Autodesk Inventor part; units mm, degrees
ref_plane "Work Plane1" through (0, 0, 7.9375) normal (0, 0, 1) x (1, 0, 0)
ref_plane "Work Plane2" through (24.3078, 0, 0) normal (1, 0, 0) x (0, 1, 0)
ref_plane "XZ Plane" through (0, 0, 0) normal (0, 1, 0) x (-1, 0, 0)
sketch "Sketch1" plane through (0, 0, 0) normal (0, 0, 1) x (1, 0, 0)
  line L0 (1.9155, 84.5388) -> (46.3655, 84.5388) construction
  line L1 (46.3655, 84.5388) -> (46.3655, 1.9888) construction
  line L2 (46.3655, 1.9888) -> (1.9155, 1.9888) construction
  line L3 (1.9155, 1.9888) -> (1.9155, 84.5388) construction
  line L4 (13.0242, 66.1379) -> (35.273, 66.1379)
  line L5 (13.0242, 66.1379) -> (13.304, 71.2552)
  line L6 (13.304, 71.2552) -> (14.5683, 76.0081)
  line L7 (14.5683, 76.0081) -> (16.9096, 79.3562)
  line L8 (16.9096, 79.3562) -> (20.1875, 81.1824)
  line L9 (20.1875, 81.1824) -> (24.3082, 82.0721)
  line L10 (24.3082, 82.0721) -> (24.3082, 66.1379)
  line L11 (35.5922, 66.1379) -> (35.3124, 71.2552)
  line L12 (35.3124, 71.2552) -> (34.0481, 76.0081)
  line L13 (34.0481, 76.0081) -> (31.7068, 79.3562)
  line L14 (31.7068, 79.3562) -> (28.4289, 81.1824)
  line L15 (28.4289, 81.1824) -> (24.3082, 82.0721)
  point P0 (0, 0)
revolve "Revolution1" add sketch "Sketch1" angle 360 about axis through (24.3082, 82.0721, 0) along (0, -1, 0)
fillet "Fillet1" radius 0.635 5 edges at (35.5922, 66.1379, 0) (35.3124, 71.2552, 0) (34.0481, 76.0081, 0) (31.7068, 79.3562, 0) (28.4289, 81.1824, 0)
ref_plane "Work Plane1" through (0, 0, 7.9375) normal (0, 0, 1) x (1, 0, 0)
sketch "Sketch2" plane through (0, 0, 7.9375) normal (0, 0, 1) x (1, 0, 0)
  line L0 (1.9442, 84.5823) -> (46.3942, 84.5823) construction
  line L1 (46.3942, 84.5823) -> (46.3942, 2.0323) construction
  line L2 (46.3942, 2.0323) -> (1.9442, 2.0323) construction
  line L3 (1.9442, 2.0323) -> (1.9442, 84.5823) construction
  circle A0 centre (18.1243, 71.3329) radius 4.1255
  circle A1 centre (30.3101, 71.3329) radius 4.1275
  line L4 (18.1243, 71.3329) -> (30.3101, 71.3329)
  line L5 (30.3101, 71.3329) -> (34.4376, 71.3329)
  line L6 (18.1243, 71.3329) -> (13.9988, 71.3329)
  point P0 (0, 0)
  point P1 (26.1826, 71.3329)
  point P2 (22.2498, 71.3329)
  dimension "d11" = 8.251
  dimension "d12" = 8.255
revolve "Revolution2" cut sketch "Sketch2" angle 360 about axis through (18.1243, 71.3329, 7.9375) along (1, 0, 0) picked at (15.4139, 71.662) picked at (28.062, 72.8846) contours L4 L6 A0 | A1 L5 L4
ref_plane "Work Plane2" through (24.3078, 0, 0) normal (1, 0, 0) x (0, 1, 0)
sketch "Sketch3" plane through (24.3078, 0, 0) normal (1, 0, 0) x (0, 1, 0)
  line L0 (83.2138, 13.5179) -> (83.2138, -13.8458) construction
  line L1 (83.2138, -13.8458) -> (60.6921, -13.8458) construction
  line L2 (60.6921, -13.8458) -> (60.6921, 13.5179) construction
  line L3 (60.6921, 13.5179) -> (83.2138, 13.5179) construction
  circle A0 centre (66.0006, -11.3657) radius 0.762
  circle A1 centre (66.0006, -11.3657) radius 0.381
  line L4 (66.1379, -10.6133) -> (66.1379, 10.6133)
  line L5 (66.6605, -11.7467) -> (67.213, -11.2252)
  line L6 (71.1899, -11.0078) -> (66.8076, -11.2474)
  line L7 (66.1379, -10.0536) -> (66.1379, -10.6133)
  line L8 (67.213, -11.2252) -> (66.7496, -11.2252)
  line L9 (65.5576, -10.7458) -> (66.1379, -10.0864)
  line L10 (66.1379, -10.0864) -> (66.1379, -10.6162)
  arc A2 (67.213, -11.2252) -> (66.1379, -10.0864) centre (66.6755, -10.6558) ccw
  point P0 (0, 0)
  dimension "d19" = 1.524
  dimension "d20" = 0.762
extrude "Extrusion1" add sketch "Sketch3" along normal mid plane 1.143
properties part number "Head_3DPrint"
The listing builds one solid part. Answer for the finished solid, in the listing's coordinates (mm). Round coordinates to 2 decimals unless told otherwise and drop trailing zeros. Loops run counter-clockwise (first coordinate to the right, second up) from the corner with the lowest first, then second, coordinate; pieces in that order, holes last. Notation, with made-up numbers: (74, 84.25) -> (89, 84.25) arc R25 cw to (89, 100.25) -> close; hole circle Ø11 at (68.5, 30.5). An arc over 180 degrees is marked (long way). Use one line per item in the form item = value.
1. The part is cut by section B-B on y = 73.5. Determine the outline of the cut face in (x, z), and give its area (3 significant figures).
Answer key:
outline = (15.52, 5.58) arc R10.41 ccw (long way) to (33.02, 5.7) arc R3.51 cw to (27.42, 9.93) arc R10.41 ccw to (21.05, 9.88) arc R3.51 cw to start
area = 299 mm²
2. The part is cut by section A-A on z = 5. Give the number of separate pieces and of enclosed holes in the cut face, and give its area (3 significant figures).
Answer key:
separate_pieces = 1
enclosed_holes = 2
area = 191 mm²
3. Flat-ended cylindrical pins translate along their axes: pin 1 Ø1.5 at (x, z) = (32, 2.5) entering from +Y; pin 2 Ø1 at (y, z) = (66, -11.5) entering from -X; pin 3 Ø8 at (x, y) = (17, 79) entering from -Z. Find the tip coordinate at first contact, or state that the pin passes through.
Answer key:
pin_1 = 79.38
pin_2 = 23.74
pin_3 = -8.54
4. Find the intervals of material crossed by probe 1 along Z at (x, y) = (22.5, 68.5); probe 2 along Y at (x, z) = (21.5, 8.25); probe 3 along X at (y, z) = (76, 2.25), in increasing order. Write a range as [from, to].
Answer key:
probe_1 = [-11.01, 11.01]
probe_2 = [66.14, 68.98], [73.68, 77.47]
probe_3 = [14.84, 33.78]
